Print and shaded views of the part. All mm, measured from the part's lowest x, y and z. Round coordinates to 2 decimals unless told otherwise and drop trailing zeros. Write each loop counter-clockwise with the first axis right and the second up, starting at its lowest first coordinate (ties: lowest second). Pieces come first, ordered by that corner, then holes.
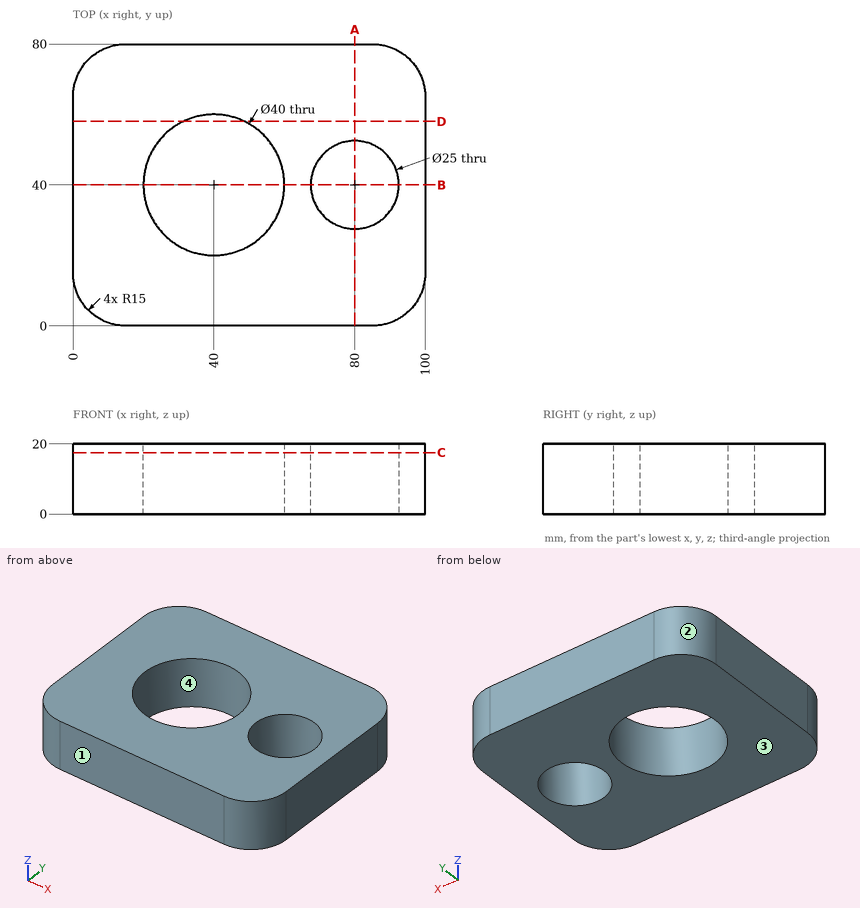
1) Slice it at A-A (x = 80). Write the cut outline in (y, z), plus the area to 3 significant figures.
Results:
outline: (0, 0) - (27.5, 0) - (27.5, 20) - (0, 20) - close; (52.5, 0) - (80, 0) - (80, 20) - (52.5, 20) - close
area: 1,100 mm2
2) Slice it at D-D (y = 58). Write the cut outline in (x, z), plus the area to 3 significant figures.
Results:
outline: (0, 0) - (31.28, 0) - (31.28, 20) - (0, 20) - close; (48.72, 0) - (100, 0) - (100, 20) - (48.72, 20) - close
area: 1,650 mm2
3) Pin check, flat tip, straight feed: pin 1 Ø15 at (x, y) = (80, 40) entering from -Z. Stop position of the tip, or through.
Results:
pin 1: passes through
4) Slice it at B-B (y = 40). Write the cut outline in (x, z), plus the area to 3 significant figures.
Results:
outline: (0, 0) - (20, 0) - (20, 20) - (0, 20) - close; (60, 0) - (67.5, 0) - (67.5, 20) - (60, 20) - close; (92.5, 0) - (100, 0) - (100, 20) - (92.5, 20) - close
area: 700 mm2
5) Wall check: L1, parallel to Y at x = 39.5, z = 12.25; L2, parallel to Y at x = 80, z = 9.75; L3, parallel to X at y = 26.5, z = 5. Give the ranges that are in metal, low to high.
Results:
L1: y = 0 to 20.01, 59.99 to 80
L2: y = 0 to 27.5, 52.5 to 80
L3: x = 0 to 25.24, 54.76 to 100
6) Mould opens along Y. For the marked faces 1, 2, 3 and 4 say: released by +Y, released by -Y, zero draft, split by the parting line, or undercut.
Results:
face 1: released by -Y
face 2: released by +Y
face 3: zero draft
face 4: undercut
7) Slice it at C-C (z = 17.5). Write the cut outline in (x, y).
Results:
outline: (0, 15) arc R15 ccw to (15, 0) - (85, 0) arc R15 ccw to (100, 15) - (100, 65) arc R15 ccw to (85, 80) - (15, 80) arc R15 ccw to (0, 65) - close; hole circle Ø40 at (40, 40); hole circle Ø25 at (80, 40)
